For this review, use the dimensioned drawing (mm, ordinates from the lowest corner) and the shaded views. A direction names the side the tool comes from. Coordinates: 2 decimals unless noted, no trailing zeros. Loops run counter-clockwise (first coordinate to the right, second up) from the corner with the lowest first, then second, coordinate; pieces in that order, holes last. Notation, with made-up numbers: (25, 5) -> (38, 5) arc R29 cw to (38, 37) -> close; hole circle Ø2 at (3, 50). An arc over 180 degrees is marked (long way). Answer as a JSON object with one key per item and string values.
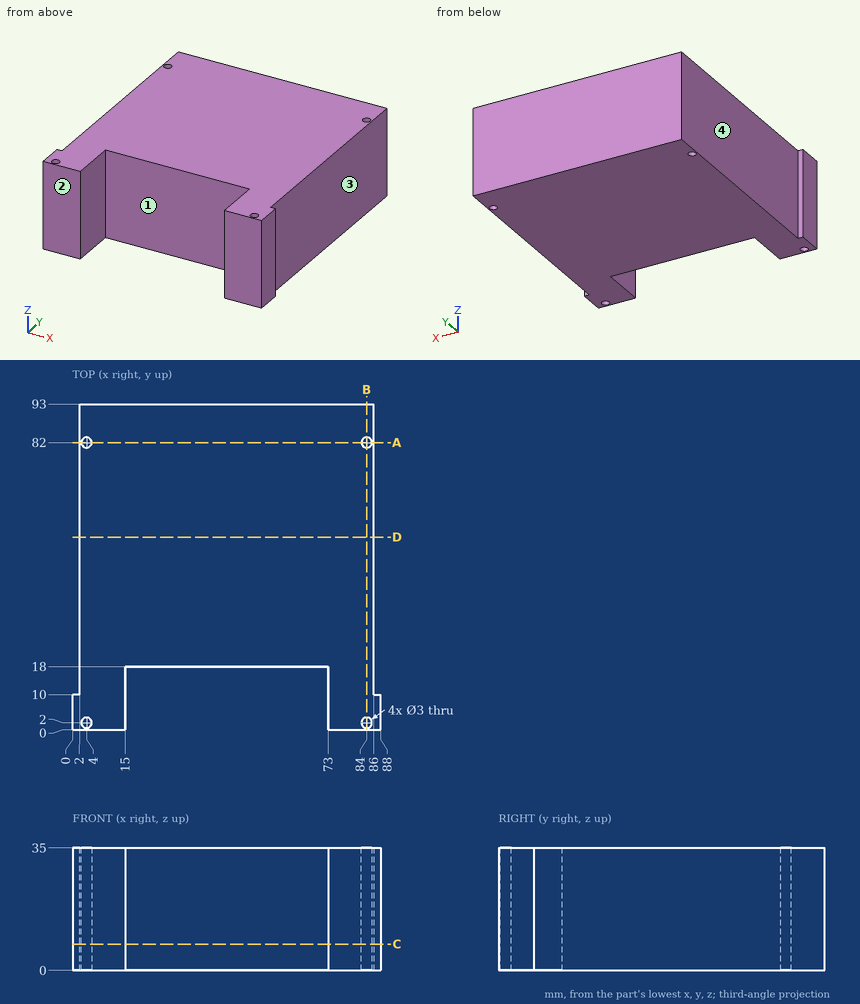
1) Add section C-C, the plane z = 7.5. Give the boundary of the cut face in (x, y).
Completed:
{"outline": "(0, 0) -> (15, 0) -> (15, 18) -> (73, 18) -> (73, 0) -> (88, 0) -> (88, 10) -> (86, 10) -> (86, 93) -> (2, 93) -> (2, 10) -> (0, 10) -> close; hole circle Ø3 at (4, 2); hole circle Ø3 at (4, 82); hole circle Ø3 at (84, 2); hole circle Ø3 at (84, 82)"}
2) Clearance check with flat-ended pins moving along their axes: pin 1 Ø10 at (y, z) = (48.5, 27) entering from -X; pin 2 Ø1 at (x, z) = (87, 21) entering from +Y; pin 3 Ø2.5 at (x, y) = (84, 2) entering from +Z; pin 4 Ø17.5 at (y, z) = (47.5, 14.5) entering from +X. State where each tip first meets the part, or that it passes through.
Completed:
{"pin 1": "x = 2", "pin 2": "y = 10", "pin 3": "through", "pin 4": "x = 86"}
3) For the marked faces 1, 2, 3 and 4, list the 3-axis set-ups (+Z, -Z, +X, -X, +Y, -Y) from which the entire face can be reached by the end or side of a thin tool; tool diameter is ignored.
Completed:
{"face 1": "+Z, -Z, -Y", "face 2": "+Z, -Z, +X, -X, -Y", "face 3": "+Z, -Z, +X, +Y", "face 4": "+Z, -Z, -X, +Y"}
4) Wall thickness on probe 1 along Y at (x, z) = (84, 22); probe 2 along X at (y, z) = (82, 21.5); probe 3 along X at (y, z) = (8.5, 18): over which ranges is each line inside the solid? List them lowest first.
Completed:
{"probe 1": "0 to 0.5, 3.5 to 80.5, 83.5 to 93", "probe 2": "2 to 2.5, 5.5 to 82.5, 85.5 to 86", "probe 3": "0 to 15, 73 to 88"}
5) Add section D-D, the plane y = 55. Give the boundary of the cut face in (x, z).
Completed:
{"outline": "(2, 0) -> (86, 0) -> (86, 35) -> (2, 35) -> close"}
6) Add section A-A, the plane y = 82. Give the boundary of the cut face in (x, z).
Completed:
{"outline": "(2, 0) -> (2.5, 0) -> (2.5, 35) -> (2, 35) -> close; (5.5, 0) -> (82.5, 0) -> (82.5, 35) -> (5.5, 35) -> close; (85.5, 0) -> (86, 0) -> (86, 35) -> (85.5, 35) -> close"}
7) Add section B-B, the plane x = 84. Give the boundary of the cut face in (y, z).
Completed:
{"outline": "(0, 0) -> (0.5, 0) -> (0.5, 35) -> (0, 35) -> close; (3.5, 0) -> (80.5, 0) -> (80.5, 35) -> (3.5, 35) -> close; (83.5, 0) -> (93, 0) -> (93, 35) -> (83.5, 35) -> close"}
